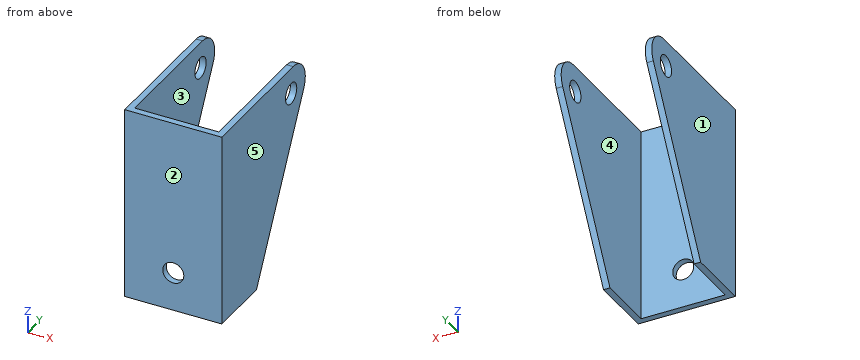
from build123d import *

# Parameters (mm, degrees)
EXTRUDE_1_DEPTH     = 60
SKETCH_2_R          = 3.25
CUT_EXTRUDE_1_DEPTH = 31
FILLET_1_R          = 7
SKETCH_3_R          = 3.25
CUT_EXTRUDE_2_DEPTH = 3


with BuildPart() as part:
    # 草图1 → 凸台-拉伸1 (new body)
    with BuildSketch(Plane.XY):
        Polygon((-13, -20.797836643), (-13, -73.797836643), (13, -73.797836643), (13, -20.797836643), (15, -20.797836643), (15, -75.797836643), (-15, -75.797836643), (-15, -20.797836643), align=None)
    extrude(amount=EXTRUDE_1_DEPTH)

    # 草图2 → 切除-拉伸1 (cut, through all)
    with BuildSketch(Plane(origin=(15, 0, 0), x_dir=(0, 0, -1), z_dir=(1, 0, 0))):
        with Locations((-52, -35.797836643)):
            Circle(SKETCH_2_R)
        Polygon((-60, -20.797836643), (-60, -22.797836643), (0, -55.797836643), (0, -20.797836643), align=None)
    extrude(amount=-CUT_EXTRUDE_1_DEPTH, mode=Mode.SUBTRACT)

    # 圆角1
    fillet_1_edges = [part.edges().sort_by_distance(p)[0] for p in [
        (14, -22.797836643, 60),
        (-14, -22.797836643, 60),
    ]]
    fillet(fillet_1_edges, radius=FILLET_1_R)

    # 草图3 → 切除-拉伸2 (cut, through all)
    with BuildSketch(Plane(origin=(0, -73.797836643, 0), x_dir=(1, 0, 0), z_dir=(0, 1, 0))):
        with Locations((0, -12)):
            Circle(SKETCH_3_R)
    extrude(amount=-CUT_EXTRUDE_2_DEPTH, mode=Mode.SUBTRACT)


solid = part.part
Geometry: final body of the model. Coordinates: model frame, mm. Face numbers are marked on the shaded views. A direction names the side the tool comes from. Round coordinates to 2 decimals unless told otherwise and drop trailing zeros. Order: outer loops, then holes, each group sorted by start corner. A loop starts at its lowest first (then second) coordinate and runs counter-clockwise, first axis right, second up.
Q1. Section B-B, the plane y = -71. Output: boundary loops of the cut face in (x, z).
Result sheet:
outline: (-15, 0) - (-13, 0) - (-13, 60) - (-15, 60) - close; (13, 0) - (15, 0) - (15, 60) - (13, 60) - close
Q2. Access query for the marked faces 4 and 5. Directions: +Z, -Z, +X, -X, +Y, -Y. A direction counts if a zero-diameter tool reaches every point of the face in a straight line with its end or side. Return the directions, or none.
Result sheet:
face 4: +Z, -Z, +Y
face 5: +Z, -Z, +X, +Y, -Y
Q3. Mould query, pull axis X, two halves, no side actions, for the marked faces 1, 2 and 3. Classes: released by +X, released by -X, zero draft, split by the parting line, or undercut.
Result sheet:
face 1: released by -X
face 2: zero draft
face 3: undercut
Q4. Section D-D, the plane z = 52. Output: boundary loops of the cut face in (x, y).
Result sheet:
outline: (-15, -75.8) - (15, -75.8) - (15, -39.05) - (13, -39.05) - (13, -73.8) - (-13, -73.8) - (-13, -39.05) - (-15, -39.05) - close; (-15, -32.55) - (-13, -32.55) - (-13, -27.71) - (-15, -27.71) - close; (13, -32.55) - (15, -32.55) - (15, -27.71) - (13, -27.71) - close
Q5. Material intervals for probe 1 along Z at (x, y) = (0, -74.25); probe 2 along X at (y, z) = (-51, 18.5); probe 3 along Y at (x, z) = (10, 47), sorted ascending.
Result sheet:
probe 1: z = 0 to 8.75, 15.25 to 60
probe 2: x = -15 to -13, 13 to 15
probe 3: y = -75.8 to -73.8
Q6. Pin query (flat end, axial travel): pin 1 (13 mm diameter, centred on x = -2, z = 27, fed in from +Y). Return the tip coordinate at first contact, or that it passes through.
Result sheet:
pin 1: stops at y = -73.8
Q7. Section A-A, the plane x = 0. Output: boundary loops of the cut face in (y, z).
Result sheet:
outline: (-75.8, 0) - (-73.8, 0) - (-73.8, 8.75) - (-75.8, 8.75) - close; (-75.8, 15.25) - (-73.8, 15.25) - (-73.8, 60) - (-75.8, 60) - close
Q8. Section C-C, the plane z = 12. Output: boundary loops of the cut face in (x, y).
Result sheet:
outline: (-15, -75.8) - (-3.25, -75.8) - (-3.25, -73.8) - (-13, -73.8) - (-13, -49.2) - (-15, -49.2) - close; (3.25, -75.8) - (15, -75.8) - (15, -49.2) - (13, -49.2) - (13, -73.8) - (3.25, -73.8) - close
